Geometry: final body of the model. Coordinates: model frame, mm. Give positions to 0.01 mm unless a question says otherwise; leave off trailing zeros. Write each loop counter-clockwise with the first axis right and the second up, starting at its lowest first coordinate (ties: lowest second). Pieces come first, ordered by that corner, then holes. Notation, with made-up numbers: M 85.25,76 L 139.25,76 A38 ccw 139.25,115 Z; hole C -38.5,41.5 d4. An arc over 180 degrees is marked long. Use a Markdown table: item, result. Add a question column.
1) Pin query (flat end, axial travel): pin 1 (19 mm diameter, centred on x = 90, z = 0, fed in from -Y); pin 2 (6 mm diameter, centred on x = 38, z = -13, fed in from +Y). Return the tip coordinate at first contact, or that it passes through.
2) Line query: line 1 (X direction, y = -0.25, z = -6.5); line 2 (X direction, y = -0.05, z = 5); line 3 (Z direction, x = 90, y = -0.7). Output: solid intervals per line, ascending.
3) Section C-C on x = 96. Return the cut outline in (y, z), then the cut area to 3 significant figures.
4) Section A-A on y = -0.75. Return the cut outline in (x, z), then the cut area to 3 significant figures.
5) Draft query along X for faces 1 (the cylindrical face through (-80.234, -0.493, 16.084)), 2 (the cylindrical face through (78.01, -0.49, 0.53)), 3 (the flat face through (11, 0, 0)). Return one class per face: +X half, -X half, draft (parallel to the pull), parting line (faces both ways), or undercut.
6) Section D-D on z = 9.5. Return the cut outline in (x, y), then the cut area to 3 significant figures.
7) Section B-B on z = -6. Return the cut outline in (x, y), then the cut area to 3 significant figures.
```python
from build123d import *

# Parameters (mm, degrees)
F0_R     = 12
F1_DEPTH = 1
F3_DEPTH = 1


with BuildPart() as f1:
    # F0 (on Front) → F1 (new body)
    with BuildSketch(Plane.XZ):
        with BuildLine():
            Line((90, 22.5), (0, 22.5))
            Line((0, 22.5), (-64.5, 22.5))
            ThreePointArc((-64.5, 22.5), (-87, 0), (-64.5, -22.5))
            Line((-64.5, -22.5), (0, -22.5))
            Line((0, -22.5), (90, -22.5))
            ThreePointArc((90, -22.5), (112.5, 0), (90, 22.5))
        make_face()
        with Locations((-64.5, 0)):
            Circle(F0_R, mode=Mode.SUBTRACT)
        with Locations((90, 0)):
            Circle(F0_R, mode=Mode.SUBTRACT)
    extrude(amount=F1_DEPTH)

    # F2 (on face) → F3 (join)
    with BuildSketch(Plane.XZ.offset(1)):
        Polygon((-84.272794, -1.934636), (-87, 0), (-87, -22.5), (-64.5, -22.5), (-70.418127, -18.801184), (-80.156557, -10.970287), align=None)
    extrude(amount=-F3_DEPTH)


solid = f1.part
```
Found:
| question | item | result |
|---|---|---|
| 1 | pin 1 | through |
| 1 | pin 2 | y = 0 |
| 2 | line 1 | -87 to -74.59, -54.41 to 79.91, 100.09 to 111.54 |
| 2 | line 2 | -86.44 to -75.41, -53.59 to 79.09, 100.91 to 111.94 |
| 2 | line 3 | -22.5 to -12, 12 to 22.5 |
| 3 | outline | M -1,-21.69 L 0,-21.69 L 0,-10.39 L -1,-10.39 Z; M -1,10.39 L 0,10.39 L 0,21.69 L -1,21.69 Z |
| 3 | area | 22.6 mm² |
| 4 | outline | M -87,-22.5 L 90,-22.5 A22.5 ccw 90,22.5 L -64.5,22.5 A22.5 ccw -87,0 Z; hole C -64.5,0 d24; hole C 90,0 d24 |
| 4 | area | 7,750 mm² |
| 5 | face 1 | -X half |
| 5 | face 2 | undercut |
| 5 | face 3 | draft |
| 6 | outline | M -84.9,-1 L -71.83,-1 L -71.83,0 L -84.9,0 Z; M -57.17,-1 L 82.67,-1 L 82.67,0 L -57.17,0 Z; M 97.33,-1 L 110.4,-1 L 110.4,0 L 97.33,0 Z |
| 6 | area | 166 mm² |
| 7 | outline | M -87,-1 L -74.89,-1 L -74.89,0 L -87,0 Z; M -54.11,-1 L 79.61,-1 L 79.61,0 L -54.11,0 Z; M 100.39,-1 L 111.69,-1 L 111.69,0 L 100.39,0 Z |
| 7 | area | 157 mm² |
